Autodesk Inventor part; units mm, degrees
ref_plane "YZ Plane" through (0, 0, 0) normal (1, 0, 0) x (0, 1, 0)
ref_plane "XZ Plane" through (0, 0, 0) normal (0, 1, 0) x (-1, 0, 0)
ref_plane "XY Plane" through (0, 0, 0) normal (0, 0, 1) x (1, 0, 0)
sketch "Sketch1" plane through (0, 0, 0) normal (0, 0, 1) x (1, 0, 0)
  line L0 (0, 0) -> (8, 0)
  line L1 (8, 0) -> (8, -1.5)
  line L2 (8, -1.5) -> (5.5711, -1.5)
  line L3 (0, -1.5) -> (0, 0)
  line L4 (0, 0) -> (5, 0) construction
  line L5 (4.2426, -2.8284) -> (5.5711, -1.5)
  line L6 (6.5, -14.0858) -> (6.5, -7.9142)
  line L7 (7.9142, -6.5) -> (15.5, -6.5)
  line L8 (0, -8) -> (1.5, -8)
  line L9 (1.5, -8) -> (1.5, -5.5711)
  line L10 (11, -11) -> (10.2929, -10.2929) construction
  line L11 (11, -11) -> (10.2929, -11.7071) construction
  line L12 (0, 0) -> (8, 0)
  line L13 (5.5711, -1.5) -> (4.2426, -2.8284)
  line L14 (2.8284, -4.2426) -> (1.5, -5.5711)
  line L15 (7.9142, -6.5) -> (4.2426, -2.8284)
  line L16 (6.5, -7.9142) -> (2.8284, -4.2426)
  circle A0 centre (11, -11) radius 2
  line L17 (11, -11) -> (16.6687, -11) construction
  line L18 (11, -16.9105) -> (11, -11) construction
  line L19 (22, 0) -> (14, 0)
  line L20 (14, 0) -> (14, -1.5)
  line L21 (14, -1.5) -> (16.4289, -1.5)
  line L22 (22, -1.5) -> (22, 0)
  line L23 (22, 0) -> (17, 0)
  line L24 (17.7574, -2.8284) -> (16.4289, -1.5)
  line L25 (15.5, -15.5) -> (15.5, -7.9142)
  line L26 (15.5, -6.5) -> (7.9142, -6.5)
  line L27 (22, -8) -> (20.5, -8)
  line L28 (20.5, -8) -> (20.5, -5.5711)
  line L29 (11, -11) -> (11.7071, -10.2929) construction
  line L30 (11, -11) -> (11.7071, -11.7071) construction
  line L31 (22, 0) -> (14, 0)
  line L32 (16.4289, -1.5) -> (17.7574, -2.8284)
  line L33 (19.1716, -4.2426) -> (20.5, -5.5711)
  line L34 (14.0858, -6.5) -> (17.7574, -2.8284)
  line L35 (15.5, -7.9142) -> (19.1716, -4.2426)
  circle A1 centre (11, -11) radius 2
  line L36 (0, -22) -> (8, -22)
  line L37 (8, -22) -> (8, -20.5)
  line L38 (8, -20.5) -> (5.5711, -20.5)
  line L39 (0, -20.5) -> (0, -22)
  line L40 (0, -22) -> (5, -22) construction
  line L41 (4.2426, -19.1716) -> (5.5711, -20.5)
  line L42 (6.5, -7.9142) -> (6.5, -14.0858)
  line L43 (6.5, -15.5) -> (14.0858, -15.5)
  line L44 (0, -14) -> (1.5, -14)
  line L45 (1.5, -14) -> (1.5, -16.4289)
  line L46 (11, -11) -> (10.2929, -11.7071) construction
  line L47 (11, -11) -> (10.2929, -10.2929) construction
  line L48 (0, -22) -> (8, -22)
  line L49 (5.5711, -20.5) -> (4.2426, -19.1716)
  line L50 (2.8284, -17.7574) -> (1.5, -16.4289)
  line L51 (7.9142, -15.5) -> (4.2426, -19.1716)
  line L52 (6.5, -14.0858) -> (2.8284, -17.7574)
  circle A2 centre (11, -11) radius 2
  line L53 (22, -22) -> (14, -22)
  line L54 (14, -22) -> (14, -20.5)
  line L55 (14, -20.5) -> (16.4289, -20.5)
  line L56 (22, -20.5) -> (22, -22)
  line L57 (22, -22) -> (17, -22)
  line L58 (17.7574, -19.1716) -> (16.4289, -20.5)
  line L59 (20.5, -14) -> (20.5, -16.4289)
  line L60 (15.5, -14.0858) -> (19.1716, -17.7574)
  line L61 (19.1716, -17.7574) -> (20.5, -16.4289)
  line L62 (14.0858, -15.5) -> (17.7574, -19.1716)
  line L63 (16.4289, -20.5) -> (17.7574, -19.1716)
  line L64 (22, -22) -> (14, -22)
  line L65 (22, -14) -> (20.5, -14)
  line L66 (11, -11) -> (11.7071, -11.7071) construction
  line L67 (11, -11) -> (11.7071, -10.2929) construction
  line L68 (14.0858, -15.5) -> (6.5, -15.5)
  line L69 (15.5, -7.9142) -> (15.5, -15.5)
  circle A3 centre (11, -11) radius 2
  line L70 (22, -14) -> (22, -20.5)
  line L71 (22, -1.5) -> (22, -8)
  line L72 (8, 0) -> (0, 0) construction
  line L73 (0, 0) -> (0, -8) construction
  line L74 (9.5858, -11) -> (9.0681, -11.5176)
  line L75 (6.5, -14.0858) -> (2.8284, -17.7574)
  line L76 (0, -22) -> (0, -14)
  line L77 (0, -8) -> (0, 0)
  line L78 (0, 0) -> (2, 0) construction
  line L79 (2, 0) -> (2, -2) construction
  circle A4 centre (2, -2) radius 1
  circle A5 centre (20, -2) radius 1
  circle A6 centre (2, -20) radius 1
  circle A7 centre (20, -20) radius 1
  point P0 (3.5355, -3.5355)
  point P1 (0, -7.0711)
  point P2 (6.5, -6.5)
  point P3 (6.5, -15.5)
  point P4 (1.5, 0)
  point P5 (10.2929, -10.2929)
  point P6 (18.4645, -3.5355)
  point P7 (22, -7.0711)
  point P8 (6.5, -6.5)
  point P9 (20.5, 0)
  point P10 (11.7071, -10.2929)
  point P11 (12.4142, -11)
  point P12 (3.5355, -18.4645)
  point P13 (0, -14.9289)
  point P14 (6.5, -6.5)
  point P15 (1.5, -22)
  point P16 (10.2929, -11.7071)
  point P17 (18.4645, -18.4645)
  point P18 (20.5, -22)
  point P19 (22, -14.9289)
  point P20 (15.5, -6.5)
  point P21 (11.7071, -11.7071)
  dimension "d2" = 8
  dimension "d3" = 1.5
  dimension "d4" = 5
  dimension "d10" = 9
  dimension "d11" = 9
  dimension "d14" = 4
  dimension "d15" = 2
  dimension "d16" = 2
  dimension "d17" = 2
extrude "Extrusion1" add sketch "Sketch1" along normal blind 300
properties part number "extrusion_300"
The model under review builds one solid part; all positions refer to its coordinate system, in mm. Round coordinates to 2 decimals unless told otherwise and drop trailing zeros. Write each question's results on one line, items separated by ' | '. Start each with the question number.
Q1. Insertion check: P1, Ø3, axis at x = 18, y = -14, coming from the +Z side. The pin has a flat end and moves straight along its axis. Give the tip position at first contact, or say it passes through.
Q2. Wall thickness on line 1 along Y through (x, z) = (11, 142); line 2 along X through (y, z) = (-5.25, 37.5); line 3 along X through (y, z) = (-5, 52): over which ranges is each line inside the solid? List them lowest first. Write a range as [from, to].
Q3. Draft analysis for pull direction Y (two halves, no side actions). For faces 1 (the flat face through (6.5, -11, 148)), 2 (the flat face through (0, -18, 148)), 3 (the flat face through (4, -22, 148)), 4 (the flat face through (15.5, -11, 148)), state which applies: pulls with the +Y half, pulls with the -Y half, needs draft (parallel to the pull), parting line crosses it, or undercut.
Q4. Take a section at A-A on z = 84. Give the number of separate pieces and of enclosed holes in the cut face, plus the area to 3 significant figures.
Data:
1) P1: passes through
2) line 1: y = [-15.5, -13], [-9, -6.5] | line 2: x = [0, 1.82], [3.84, 6.66], [15.34, 18.16], [20.18, 22] | line 3: x = [0, 2.07], [3.59, 6.41], [15.59, 18.41], [19.93, 22]
3) face 1: undercut | face 2: needs draft | face 3: pulls with the -Y half | face 4: undercut
4) separate pieces: 1 | enclosed holes: 5 | area: 214 mm²
